from build123d import *

# Parameters (mm, degrees)
SKETCH1_R           = 11
BOSS_EXTRUDE1_DEPTH = 2.25
SKETCH2_R           = 8
BOSS_EXTRUDE2_DEPTH = 2.25
BOSS_EXTRUDE3_DEPTH = 2.25
SKETCH4_R           = 4.8
CUT_EXTRUDE1_DEPTH  = 4.5


with BuildPart() as part:
    # Sketch1 → Boss-Extrude1 (new, symmetric)
    with BuildSketch(Plane.XY):
        Circle(SKETCH1_R)
    extrude(amount=BOSS_EXTRUDE1_DEPTH, both=True)



with BuildPart() as body_2:
    # Sketch2 → Boss-Extrude2 (new, symmetric)
    with BuildSketch(Plane.XY):
        with Locations((66.0482, 0)):
            Circle(SKETCH2_R)
    extrude(amount=BOSS_EXTRUDE2_DEPTH, both=True)


with BuildPart() as part_1:
    add(part.part)

    add(body_2.part)  # Boss-Extrude3 merges body 2
    # Sketch3 → Boss-Extrude3 (add, symmetric)
    with BuildSketch(Plane.XY):
        Polygon((0, -9), (66.0482, -6.5), (66.0482, 6.5), (0, 9), align=None)
    extrude(amount=BOSS_EXTRUDE3_DEPTH, both=True)

    # Sketch4 → Cut-Extrude1 (cut, symmetric)
    with BuildSketch(Plane.XY):
        Circle(SKETCH4_R)
        with Locations((66.0482, 0)):
            Circle(SKETCH4_R)
    extrude(amount=CUT_EXTRUDE1_DEPTH, both=True, mode=Mode.SUBTRACT)


solid = part_1.part
Input: part model. Units: mm. Frame: model coordinates. A direction names the side the tool comes from. Give positions to 0.01 mm unless a question says otherwise; leave off trailing zeros. Order: outer loops, then holes, each group sorted by start corner. A loop starts at its lowest first (then second) coordinate and runs counter-clockwise, first axis right, second up. Notation, with made-up numbers: (29, 71) - (67, 71) arc R14 ccw to (67, 87) - close; hole circle Ø7 at (34, 77). An arc over 180 degrees is marked (long way). Write each question's results on one line, items separated by ' | '.
Item 1: Section B-B (y = 0). Return loops of the section in (x, z).
A:
outline: (-11, -2.25) - (-4.8, -2.25) - (-4.8, 2.25) - (-11, 2.25) - close; (4.8, -2.25) - (61.25, -2.25) - (61.25, 2.25) - (4.8, 2.25) - close; (70.85, -2.25) - (74.05, -2.25) - (74.05, 2.25) - (70.85, 2.25) - close
Item 2: Access query for faces 1 (the flat face through (34.533, 7.693, 0.031)), 2 (the flat face through (31, 0, 2.25)). Directions: +Z, -Z, +X, -X, +Y, -Y. A direction counts if a zero-diameter tool reaches every point of the face in a straight line with its end or side. Return the directions, or none.
A:
face 1: +Z, -Z, +Y | face 2: +Z, +X, -X, +Y, -Y
Item 3: Material intervals for line 1 along Y through (x, z) = (0, -0.8); line 2 along Y through (x, z) = (-4, -1.65); line 3 along X through (y, z) = (-2.25, 2.05), sorted ascending.
A:
line 1: y = -11 to -4.8, 4.8 to 11 | line 2: y = -10.25 to -2.65, 2.65 to 10.25 | line 3: x = -10.77 to -4.24, 4.24 to 61.81, 70.29 to 73.73
Item 4: Draft query along X for faces 3 (the cylindrical face through (74.045, -0.241, 0.031)), 4 (the flat face through (31, 0, -2.25)), 5 (the cylindrical face through (-11, 0, 0)), 6 (the flat face through (33.763, -7.722, 0.031)). Return one class per face: released by +X, released by -X, zero draft, split by the parting line, or undercut.
A:
face 3: undercut | face 4: zero draft | face 5: split by the parting line | face 6: undercut
Item 5: Section A-A (x = 0). Return loops of the section in (y, z), and give its area (3 significant figures).
A:
outline: (-11, -2.25) - (-4.8, -2.25) - (-4.8, 2.25) - (-11, 2.25) - close; (4.8, -2.25) - (11, -2.25) - (11, 2.25) - (4.8, 2.25) - close | area: 55.8 mm^2
Item 6: Section C-C (z = -1.15). Return loops of the section in (x, y).
A:
outline: (6.67, -8.75) - (61.63, -6.67) arc R8 ccw (long way) to (61.63, 6.67) - (6.67, 8.75) arc R11 ccw (long way) to start; hole circle Ø9.6 at (0, 0); hole circle Ø9.6 at (66.05, 0)
Item 7: Contact query for flat-ended pins moving along their axis: pin 1 Ø2 at (x, z) = (8, -0.5) entering from +Y; pin 2 Ø6 at (x, y) = (0, 0) entering from -Z. Output: stop coordinate, or through.
A:
pin 1: stops at y = 8.74 | pin 2: passes through
Item 8: Section D-D (x = 66.5). Return loops of the section in (y, z), and give its area (3 significant figures).
A:
outline: (-7.99, -2.25) - (-4.78, -2.25) - (-4.78, 2.25) - (-7.99, 2.25) - close; (4.78, -2.25) - (7.99, -2.25) - (7.99, 2.25) - (4.78, 2.25) - close | area: 28.9 mm^2
